```python
from build123d import *

# Parameters (mm, degrees)
SKETCH_1_R      = 1.6
SKETCH_1_R_2    = 2.1
EXTRUDE_1_DEPTH = 10


with BuildPart() as part:
    # Эскиз1 → Бобышка-Вытянуть1 (new body)
    with BuildSketch(Plane(origin=(0, 0, 0), x_dir=(1, 0, 0), z_dir=(0, 1, 0))):
        with BuildLine():
            Line((-105, 110), (-89.142135624, 110))
            ThreePointArc((-89.142135624, 110), (-87.228718462, 109.619397663), (-85.606601718, 108.535533906))
            Line((-85.606601718, 108.535533906), (-58.535533906, 81.464466094))
            ThreePointArc((-58.535533906, 81.464466094), (-56.913417162, 80.380602337), (-55, 80))
            Line((-55, 80), (55, 80))
            ThreePointArc((55, 80), (56.913417162, 80.380602337), (58.535533906, 81.464466094))
            Line((58.535533906, 81.464466094), (85.606601718, 108.535533906))
            ThreePointArc((85.606601718, 108.535533906), (87.228718462, 109.619397663), (89.142135624, 110))
            Line((89.142135624, 110), (105, 110))
            ThreePointArc((105, 110), (108.535533906, 108.535533906), (110, 105))
            Line((110, 105), (110, 89.142135624))
            ThreePointArc((110, 89.142135624), (109.619397663, 87.228718462), (108.535533906, 85.606601718))
            Line((108.535533906, 85.606601718), (76.464466094, 53.535533906))
            ThreePointArc((76.464466094, 53.535533906), (75.380602337, 51.913417162), (75, 50))
            Line((75, 50), (75, 44.142135624))
            ThreePointArc((75, 44.142135624), (75.380602337, 42.228718462), (76.464466094, 40.606601718))
            Line((76.464466094, 40.606601718), (98.535533906, 18.535533906))
            ThreePointArc((98.535533906, 18.535533906), (99.619397663, 16.913417162), (100, 15))
            Line((100, 15), (100, -15))
            ThreePointArc((100, -15), (99.619397663, -16.913417162), (98.535533906, -18.535533906))
            Line((98.535533906, -18.535533906), (76.464466094, -40.606601718))
            ThreePointArc((76.464466094, -40.606601718), (75.380602337, -42.228718462), (75, -44.142135624))
            Line((75, -44.142135624), (75, -50))
            ThreePointArc((75, -50), (75.380602337, -51.913417162), (76.464466094, -53.535533906))
            Line((76.464466094, -53.535533906), (108.535533906, -85.606601718))
            ThreePointArc((108.535533906, -85.606601718), (109.619397663, -87.228718462), (110, -89.142135624))
            Line((110, -89.142135624), (110, -105))
            ThreePointArc((110, -105), (108.535533906, -108.535533906), (105, -110))
            Line((105, -110), (89.142135624, -110))
            ThreePointArc((89.142135624, -110), (87.228718462, -109.619397663), (85.606601718, -108.535533906))
            Line((85.606601718, -108.535533906), (58.535533906, -81.464466094))
            ThreePointArc((58.535533906, -81.464466094), (56.913417162, -80.380602337), (55, -80))
            Line((55, -80), (-55, -80))
            ThreePointArc((-55, -80), (-56.913417162, -80.380602337), (-58.535533906, -81.464466094))
            Line((-58.535533906, -81.464466094), (-85.606601718, -108.535533906))
            ThreePointArc((-85.606601718, -108.535533906), (-87.228718462, -109.619397663), (-89.142135624, -110))
            Line((-89.142135624, -110), (-105, -110))
            ThreePointArc((-105, -110), (-108.535533906, -108.535533906), (-110, -105))
            Line((-110, -105), (-110, -89.142135624))
            ThreePointArc((-110, -89.142135624), (-109.619397663, -87.228718462), (-108.535533906, -85.606601718))
            Line((-108.535533906, -85.606601718), (-101.464466094, -78.535533906))
            ThreePointArc((-101.464466094, -78.535533906), (-100.380602337, -76.913417162), (-100, -75))
            Line((-100, -75), (-100, -45))
            ThreePointArc((-100, -45), (-99.619397663, -43.086582838), (-98.535533906, -41.464466094))
            Line((-98.535533906, -41.464466094), (-76.464466094, -19.393398282))
            ThreePointArc((-76.464466094, -19.393398282), (-75.380602337, -17.771281538), (-75, -15.857864376))
            Line((-75, -15.857864376), (-75, 15.857864376))
            ThreePointArc((-75, 15.857864376), (-75.380602337, 17.771281538), (-76.464466094, 19.393398282))
            Line((-76.464466094, 19.393398282), (-98.535533906, 41.464466094))
            ThreePointArc((-98.535533906, 41.464466094), (-99.619397663, 43.086582838), (-100, 45))
            Line((-100, 45), (-100, 75))
            ThreePointArc((-100, 75), (-100.380602337, 76.913417162), (-101.464466094, 78.535533906))
            Line((-101.464466094, 78.535533906), (-108.535533906, 85.606601718))
            ThreePointArc((-108.535533906, 85.606601718), (-109.619397663, 87.228718462), (-110, 89.142135624))
            Line((-110, 89.142135624), (-110, 105))
            ThreePointArc((-110, 105), (-108.535533906, 108.535533906), (-105, 110))
        make_face()
        with Locations(Location((105, 105, 0), (0, 0, 270))):
            Circle(SKETCH_1_R, mode=Mode.SUBTRACT)
        with Locations(Location((105, -105, 0), (0, 0, 270))):
            Circle(SKETCH_1_R, mode=Mode.SUBTRACT)
        with Locations(Location((-105, -105, 0), (0, 0, 270))):
            Circle(SKETCH_1_R, mode=Mode.SUBTRACT)
        with Locations(Location((-105, 105, 0), (0, 0, 270))):
            Circle(SKETCH_1_R, mode=Mode.SUBTRACT)
        with Locations(Location((-91, 70, 0), (0, 0, 270))):
            Circle(SKETCH_1_R_2, mode=Mode.SUBTRACT)
        with Locations(Location((-59, 70, 0), (0, 0, 270))):
            Circle(SKETCH_1_R_2, mode=Mode.SUBTRACT)
        with Locations(Location((-59, 50, 0), (0, 0, 270))):
            Circle(SKETCH_1_R_2, mode=Mode.SUBTRACT)
        with Locations(Location((-91, 50, 0), (0, 0, 270))):
            Circle(SKETCH_1_R_2, mode=Mode.SUBTRACT)
        with Locations(Location((-59, -50, 0), (0, 0, 270))):
            Circle(SKETCH_1_R_2, mode=Mode.SUBTRACT)
        with Locations(Location((-91, -50, 0), (0, 0, 270))):
            Circle(SKETCH_1_R_2, mode=Mode.SUBTRACT)
        with Locations(Location((-91, -70, 0), (0, 0, 270))):
            Circle(SKETCH_1_R_2, mode=Mode.SUBTRACT)
        with Locations(Location((-59, -70, 0), (0, 0, 270))):
            Circle(SKETCH_1_R_2, mode=Mode.SUBTRACT)
        with Locations(Location((91, -10, 0), (0, 0, 270))):
            Circle(SKETCH_1_R_2, mode=Mode.SUBTRACT)
        with Locations(Location((59, -10, 0), (0, 0, 270))):
            Circle(SKETCH_1_R_2, mode=Mode.SUBTRACT)
        with Locations(Location((59, 10, 0), (0, 0, 270))):
            Circle(SKETCH_1_R_2, mode=Mode.SUBTRACT)
        with Locations(Location((91, 10, 0), (0, 0, 270))):
            Circle(SKETCH_1_R_2, mode=Mode.SUBTRACT)
        with Locations(Location((0, -20, 0), (0, 0, 270))):
            Circle(SKETCH_1_R, mode=Mode.SUBTRACT)
        with Locations(Location((0, 20, 0), (0, 0, 270))):
            Circle(SKETCH_1_R, mode=Mode.SUBTRACT)
        with BuildLine():
            Line((-23.535533906, -46.464466094), (-8.535533906, -31.464466094))
            ThreePointArc((-8.535533906, -31.464466094), (-6.913417162, -30.380602337), (-5, -30))
            Line((-5, -30), (5, -30))
            ThreePointArc((5, -30), (6.913417162, -30.380602337), (8.535533906, -31.464466094))
            Line((8.535533906, -31.464466094), (23.535533906, -46.464466094))
            ThreePointArc((23.535533906, -46.464466094), (24.619397663, -51.913417162), (20, -55))
            Line((20, -55), (-20, -55))
            ThreePointArc((-20, -55), (-24.619397663, -51.913417162), (-23.535533906, -46.464466094))
        make_face(mode=Mode.SUBTRACT)
        with BuildLine():
            Line((23.535533906, 46.464466094), (8.535533906, 31.464466094))
            ThreePointArc((8.535533906, 31.464466094), (6.913417162, 30.380602337), (5, 30))
            Line((5, 30), (-5, 30))
            ThreePointArc((-5, 30), (-6.913417162, 30.380602337), (-8.535533906, 31.464466094))
            Line((-8.535533906, 31.464466094), (-23.535533906, 46.464466094))
            ThreePointArc((-23.535533906, 46.464466094), (-24.619397663, 51.913417162), (-20, 55))
            Line((-20, 55), (20, 55))
            ThreePointArc((20, 55), (24.619397663, 51.913417162), (23.535533906, 46.464466094))
        make_face(mode=Mode.SUBTRACT)
        with BuildLine():
            Line((-50, 15), (-50, -15))
            ThreePointArc((-50, -15), (-46.913417162, -19.619397663), (-41.464466094, -18.535533906))
            Line((-41.464466094, -18.535533906), (-26.464466094, -3.535533906))
            ThreePointArc((-26.464466094, -3.535533906), (-25, 0), (-26.464466094, 3.535533906))
            Line((-26.464466094, 3.535533906), (-41.464466094, 18.535533906))
            ThreePointArc((-41.464466094, 18.535533906), (-46.913417162, 19.619397663), (-50, 15))
        make_face(mode=Mode.SUBTRACT)
        with BuildLine():
            Line((41.464466094, 18.535533906), (26.464466094, 3.535533906))
            ThreePointArc((26.464466094, 3.535533906), (25, 0), (26.464466094, -3.535533906))
            Line((26.464466094, -3.535533906), (41.464466094, -18.535533906))
            ThreePointArc((41.464466094, -18.535533906), (46.913417162, -19.619397663), (50, -15))
            Line((50, -15), (50, 15))
            ThreePointArc((50, 15), (46.913417162, 19.619397663), (41.464466094, 18.535533906))
        make_face(mode=Mode.SUBTRACT)
    extrude(amount=EXTRUDE_1_DEPTH)


solid = part.part
```
Check sheet for the modelled part. Datum: model origin and axes. Units: mm. A direction names the side the tool comes from. Give positions to 0.01 mm unless a question says otherwise; leave off trailing zeros. Write each loop counter-clockwise with the first axis right and the second up, starting at its lowest first coordinate (ties: lowest second). Pieces come first, ordered by that corner, then holes. Notation, with made-up numbers: (59, -0.75) - (69, -0.75) arc R17 cw to (69, 7.25) - close; hole circle Ø4 at (5, 11.5). An arc over 180 degrees is marked (long way). Answer as a JSON object with one key per item and string values. Group by question number.
1) Access from +Z, -Z, +X, -X, +Y, -Y to the whole of each face (thin tool, end or side, straight path). Record for faces 1 (the face through (100, 5, 0)), 2 (the face through (-1, 5, -80)), 3 (the face through (-16.14, 4.93, 39.07)), 4 (the face through (-75, 5, 0)).
2) Sectioned sample at B-B (y = 5.25). Give the number of separate pieces and of enclosed holes in the cut face, then the cut area to 3 significant figures.
3) Thickness scan on probe 1 along X at (y, z) = (3, -50); probe 2 along Z at (x, y) = (-23.5, 4.5); probe 3 along Z at (x, y) = (-105, 6). Record the ranges inside material, lowest first. Write a range as from..to.
4) Sectioned sample at C-C (z = 24.5). Record the cut outline in (x, y), then the cut area to 3 significant figures.
5) Release check for a two-part mould opening along Z. For faces 5 (the face through (46.989, 4.93, -19.587)), 6 (the face through (108, 5, -109)), 7 (the face through (72.26, 4.93, 95.19)) record: pulls with the +Z half, pulls with the -Z half, needs draft (parallel to the pull), parting line crosses it, or undercut.
6) Depth check by flat-ended pin: P1, Ø8, axis at x = -75, z = 12, coming from the -Y side; P2, Ø1, axis at y = 6, z = 28.5, coming from the -X side; P3, Ø2, axis at x = 49.5, y = 7.5, coming from the -Z side; P4, Ø1.8, axis at y = 2.5, z = 46, coming from the +X side. Enter the tip coordinate at first touch or a pass-through.
7) Sectioned sample at A-A (x = 45.5). Record the cut outline in (y, z).
Geometry results:
{
 "1": {"face 1": "+X, +Y, -Y", "face 2": "-Z, +Y, -Y", "face 3": "+Y, -Y", "face 4": "-X, +Y, -Y"},
 "2": {"separate pieces": "1", "enclosed holes": "22", "area": "29,800 mm^2"},
 "3": {"probe 1": "x = -100..-93.1, -88.9..-61.1, -56.9..-25, 25..75", "probe 2": "z = -80..-53.57, -46.43..46.43, 53.57..80", "probe 3": "z = -110..-106.6, -103.4..-82.07, 82.07..103.4, 106.6..110"},
 "4": {"outline": "(-81.57, 0) - (92.57, 0) - (92.57, 10) - (-81.57, 10) - close", "area": "1,740 mm^2"},
 "5": {"face 5": "undercut", "face 6": "pulls with the -Z half", "face 7": "pulls with the +Z half"},
 "6": {"P1": "stops at y = 0", "P2": "stops at x = -86.07", "P3": "stops at z = -80", "P4": "stops at x = 75"},
 "7": {"outline": "(0, -80) - (10, -80) - (10, -19.97) - (0, -19.97) - close; (0, 19.97) - (10, 19.97) - (10, 80) - (0, 80) - close"}
}
